Could you check a few things on this model? Use its own coordinates, in mm. Round coordinates to 2 decimals unless told otherwise and drop trailing zeros. Loops run counter-clockwise (first coordinate to the right, second up) from the corner with the lowest first, then second, coordinate; pieces in that order, holes last. Notation, with made-up numbers: M -31,50.25 L 18,50.25 A17 cw 18,68.25 Z; hole C 16.5,68 d5. An arc over 180 degrees is marked long. Return JSON: item names as keys, results as strings. Group by question number.
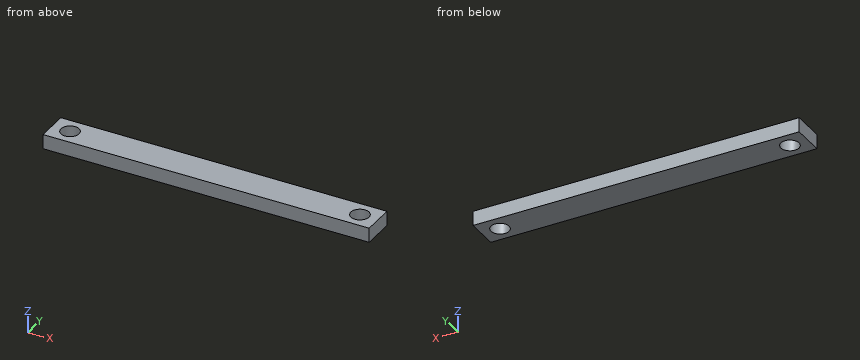
```python
from build123d import *

# Parameters (mm, degrees)
ESQUISSE1_W = 90
ESQUISSE1_H = 8.926229508
ESQUISSE1_R = 2.5
BASE_DEPTH  = 4


with BuildPart() as part:
    # Esquisse1 → BASE (new body)
    with BuildSketch(Plane.XY):
        Rectangle(ESQUISSE1_W, ESQUISSE1_H)
        with Locations((-40, 0)):
            Circle(ESQUISSE1_R, mode=Mode.SUBTRACT)
        with Locations(Location((40, 0, 0), (0, 0, 180))):
            Circle(ESQUISSE1_R, mode=Mode.SUBTRACT)
    extrude(amount=BASE_DEPTH)


solid = part.part
```
1. If we section it at A-A, the plane x = 40: Please give me the cut outline in (y, z), then the cut area to 3 significant figures.
2. If we section it at C-C, the plane z = 1.1: Please give me the cut outline in (x, y).
3. If we section it at B-B, the plane y = 0: Please give me the cut outline in (x, z).
4. I need wall thicknesses on probe 1 along Y at (x, z) = (40, 0.95); probe 2 along X at (y, z) = (-0.5, 1.2); probe 3 along X at (y, z) = (-1.5, 3.3). Which ranges of each line are inside material? Lowest first, please.
Geometry results:
{
 "1": {"outline": "M -4.46,0 L -2.5,0 L -2.5,4 L -4.46,4 Z; M 2.5,0 L 4.46,0 L 4.46,4 L 2.5,4 Z", "area": "15.7 mm^2"},
 "2": {"outline": "M -45,-4.46 L 45,-4.46 L 45,4.46 L -45,4.46 Z; hole C -40,0 d5; hole C 40,0 d5"},
 "3": {"outline": "M -45,0 L -42.5,0 L -42.5,4 L -45,4 Z; M -37.5,0 L 37.5,0 L 37.5,4 L -37.5,4 Z; M 42.5,0 L 45,0 L 45,4 L 42.5,4 Z"},
 "4": {"probe 1": "-4.46 to -2.5, 2.5 to 4.46", "probe 2": "-45 to -42.45, -37.55 to 37.55, 42.45 to 45", "probe 3": "-45 to -42, -38 to 38, 42 to 45"}
}
